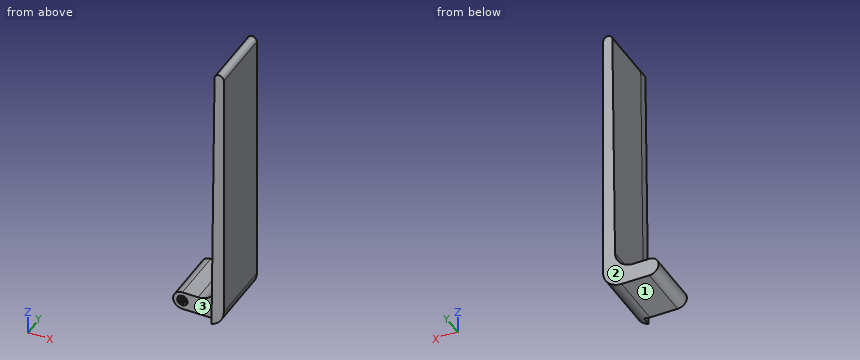
```python
from build123d import *

# Parameters (mm, degrees)
BOSS_EXTRUDE2_DEPTH = 30
FILLET1_R           = 10
FILLET2_R           = 10
SKETCH2_R           = 3.747343823
BOSS_EXTRUDE3_DEPTH = 15
BOSS_EXTRUDE4_START = 5
BOSS_EXTRUDE4_DEPTH = 5
FILLET3_R           = 10


with BuildPart() as part:
    # Sketch1 → Boss-Extrude2 (new body)
    with BuildSketch(Plane(origin=(0, 0, 0), x_dir=(1, 0, 0), z_dir=(0, 1, 0))):
        with BuildLine():
            Line((0, 5), (25, 5))
            Line((25, 5), (25, -145))
            ThreePointArc((25, -145), (22.513876781, -147.499961487), (20.000154052, -145.027753135))
            Line((20.000154052, -145.027753135), (18.445574612, -5))
            Line((18.445574612, -5), (0, -5))
            ThreePointArc((0, -5), (-5, 0), (0, 5))
        make_face()
        Polygon((0.333439775, 2.639447604), (0, 3.05), (-0.333439775, 2.639447604), (-0.758504156, 2.954178641), (-0.979368078, 2.473601404), (-1.469348706, 2.672735374), (-1.563759083, 2.15232973), (-2.087868673, 2.223354314), (-2.049893354, 1.695819264), (-2.575200173, 1.634271725), (-2.407225286, 1.132754236), (-2.900722375, 0.942501833), (-2.6133024, 0.498514094), (-3.043981522, 0.191511085), (-2.655176114, -0.167049522), (-2.995976115, -0.571513009), (-2.530215347, -0.822116802), (-2.75972251, -1.298626839), (-2.246271844, -1.42552746), (-2.35006539, -1.944143169), (-1.821186821, -1.939366985), (-1.792745019, -2.467501833), (-1.281669931, -2.33134895), (-1.122779886, -2.835818282), (-0.661621006, -2.576843686), (-0.382266362, -3.025949839), (0, -2.660425857), (0.382266362, -3.025949839), (0.661621006, -2.576843686), (1.122779886, -2.835818282), (1.281669931, -2.33134895), (1.792745019, -2.467501833), (1.821186821, -1.939366985), (2.35006539, -1.944143169), (2.246271844, -1.42552746), (2.75972251, -1.298626839), (2.530215347, -0.822116802), (2.995976115, -0.571513009), (2.655176114, -0.167049522), (3.043981522, 0.191511085), (2.6133024, 0.498514094), (2.900722375, 0.942501833), (2.407225286, 1.132754236), (2.575200173, 1.634271725), (2.049893354, 1.695819264), (2.087868673, 2.223354314), (1.563759083, 2.15232973), (1.469348706, 2.672735374), (0.979368078, 2.473601404), (0.758504156, 2.954178641), align=None, mode=Mode.SUBTRACT)
    extrude(amount=BOSS_EXTRUDE2_DEPTH)

    # Fillet1
    fillet1_edges = [part.edges().sort_by_distance(p)[0] for p in [
        (18.445574612, 15, 5),
    ]]
    fillet(fillet1_edges, radius=FILLET1_R)

    # Fillet2
    fillet2_edges = [part.edges().sort_by_distance(p)[0] for p in [
        (25, 15, -5),
    ]]
    fillet(fillet2_edges, radius=FILLET2_R)

    # Sketch2 → Boss-Extrude3 (add)
    with BuildSketch(Plane(origin=(0, 30, 0), x_dir=(1, 0, 0), z_dir=(0, 1, 0))):
        Circle(SKETCH2_R)
    extrude(amount=-BOSS_EXTRUDE3_DEPTH)

    # Sketch3 → Boss-Extrude4 (add)
    with BuildSketch(Plane.XZ.offset(BOSS_EXTRUDE4_START)):
        with BuildLine():
            Line((20.000154052, 145.027753135), (18.34093441, -4.425399581))
            Line((18.34093441, -4.425399581), (25, -4.425399581))
            Line((25, -4.425399581), (25, 145))
            ThreePointArc((25, 145), (22.513876781, 147.499961487), (20.000154052, 145.027753135))
        make_face()
    extrude(amount=-BOSS_EXTRUDE4_DEPTH)

    # Fillet3
    # the kernel refuses this fillet: 10 mm, written as the material it takes off along each edge
    with BuildSketch(Plane(origin=(25, -28.563498953, -4.425399581), x_dir=(0, 0, 1), z_dir=(0, 1, 0))) as fillet3_piece_1:
        with BuildLine():
            CenterArc((9.425399581, -10), FILLET3_R, 90, 70.482580004)
            Line((0, -6.65906559), (-0.188507992, -6.592246902))
            ThreePointArc((-0.188507992, -6.592246902), (-0.2, -3.329532795), (-0.2, 0))
            Line((-0.2, 0), (0, 0.2))
            Line((0, 0.2), (9.425399581, 0.2))
            Line((9.425399581, 0.2), (9.425399581, 0))
        make_face()
    extrude(amount=52.126997906, mode=Mode.SUBTRACT)


solid = part.part
```
Source: CAD feature listing. Evaluate the final solid. Frame: model axes, mm. Face numbers are marked on the shaded views. Round coordinates to 2 decimals unless told otherwise and drop trailing zeros. Order: outer loops, then holes, each group sorted by start corner. A loop starts at its lowest first (then second) coordinate and runs counter-clockwise, first axis right, second up. Notation, with made-up numbers: (57.25, 20) -> (100.25, 20) arc R25 ccw to (100.25, 57) -> close; hole circle Ø4 at (-23, -22). An arc over 180 degrees is marked (long way). One line per item, written item: value. Start each with the question number.
Q1. Pin query (flat end, axial travel): pin 1 (4.5 mm diameter, centred on x = 5.5, y = 10, fed in from +Z); pin 2 (10 mm diameter, centred on y = 23, z = 47.5, fed in from -X); pin 3 (8 mm diameter, centred on x = 13, z = 15.5, fed in from +Y); pin 4 (5 mm diameter, centred on y = 5, z = 35.5, fed in from -X). Return the tip coordinate at first contact, or that it passes through.
Q2. Section query A-A (y = 24.5). Return the cut outline in (x, z), plus the area to 3 significant figures.
Q3. Section query B-B (z = 111). Return the cut outline in (x, y).
Q4. Section query C-C (x = 5). Return the cut outline in (y, z), plus the area to 3 significant figures.
Q5. Material intervals for probe 1 along Z at (x, y) = (9, 1); probe 2 along X at (y, z) = (2.5, 139); probe 3 along Z at (x, y) = (12.75, 20.5), sorted ascending.
Q6. Draft query along Y for the marked faces 1, 2 and 3. Return one class per face: pulls with the +Y half, pulls with the -Y half, needs draft (parallel to the pull), parting line crosses it, or undercut.
Q7. Section query D-D (z = 17.5). Return the cut outline in (x, y).
Findings below:
1. pin 1: z = 5
1. pin 2: x = 18.86
1. pin 3: through
1. pin 4: x = 18.76
2. outline: (0, -5) -> (15, -5) arc R10 ccw to (25, 5) -> (25, 145) arc R2.5 ccw to (20, 145.03) -> (18.56, 14.89) arc R10 cw to (8.56, 5) -> (0, 5) arc R5 ccw to start
2. area: 1,110 mm²
3. outline: (19.62, -5) -> (25, -5) -> (25, 30) -> (19.62, 30) -> close
4. outline: (0, -5) -> (30, -5) -> (30, 5) -> (0, 5) -> close
4. area: 300 mm²
5. probe 1: -5 to 5.01
5. probe 2: 19.93 to 25
5. probe 3: -5 to 5.92
6. face 1: needs draft
6. face 2: pulls with the +Y half
6. face 3: pulls with the -Y half
7. outline: (18.58, -5) -> (25, -5) -> (25, 30) -> (18.58, 30) -> close
